Input: part model. Units: mm. Frame: model coordinates. Coordinates: 2 decimals unless noted, no trailing zeros. Loops run counter-clockwise (first coordinate to the right, second up) from the corner with the lowest first, then second, coordinate; pieces in that order, holes last.
```python
from build123d import *

# Parameters (mm, degrees)
SKETCH1_W                       = 558.8
SKETCH1_H                       = 25.4
BOSS_EXTRUDE1_DEPTH             = 6.35
F_1_4_0_25_DIAMETER_HOLE1_D     = 6.35
F_1_4_0_25_DIAMETER_HOLE1_DEPTH = 17.019524
F_1_4_0_25_DIAMETER_HOLE1_TIP   = 1.907732465
SKETCH5_R                       = 6.35
CUT_EXTRUDE1_DEPTH              = 280.760562803


with BuildPart() as part:
    # Sketch1 → Boss-Extrude1 (new body)
    with BuildSketch(Plane(origin=(0, 0, 0), x_dir=(1, 0, 0), z_dir=(0, 1, 0))):
        Rectangle(SKETCH1_W, SKETCH1_H)
    extrude(amount=BOSS_EXTRUDE1_DEPTH)

    # 1/4 (0.25) Diameter Hole1
    with Locations(Plane(origin=(0, 6.35, 0), x_dir=(1, 0, 0), z_dir=(0, 1, 0))):
        with Locations((-269.875, 0), (269.875, 0)):
            Hole(F_1_4_0_25_DIAMETER_HOLE1_D / 2, depth=F_1_4_0_25_DIAMETER_HOLE1_DEPTH)
            with Locations((0, 0, -(F_1_4_0_25_DIAMETER_HOLE1_DEPTH + F_1_4_0_25_DIAMETER_HOLE1_TIP / 2))):  # 118° drill point
                Cone(0, F_1_4_0_25_DIAMETER_HOLE1_D / 2, F_1_4_0_25_DIAMETER_HOLE1_TIP, mode=Mode.SUBTRACT)

    # Sketch5 → Cut-Extrude1 (cut, through all)
    with BuildSketch(Plane(origin=(0, 6.35, 0), x_dir=(1, 0, 0), z_dir=(0, 1, 0))):
        with Locations(Location((0, 0, 0), (0, 0, 270))):
            Circle(SKETCH5_R)
    extrude(amount=-CUT_EXTRUDE1_DEPTH, mode=Mode.SUBTRACT)


solid = part.part
```
Item 1: Section query A-A (x = 0). Output: boundary loops of the cut face in (y, z).
Result:
outline: (0, -12.7) - (6.35, -12.7) - (6.35, -6.35) - (0, -6.35) - close; (0, 6.35) - (6.35, 6.35) - (6.35, 12.7) - (0, 12.7) - close
Item 2: Line query: L1, parallel to X at y = 3, z = 5.5; L2, parallel to X at y = 1, z = -1; L3, parallel to X at y = 3.5, z = 4. Output: solid intervals per line, ascending.
Result:
L1: x = -279.4 to -3.17, 3.17 to 279.4
L2: x = -279.4 to -272.89, -266.86 to -6.27, 6.27 to 266.86, 272.89 to 279.4
L3: x = -279.4 to -4.93, 4.93 to 279.4
Item 3: Mould query, pull axis X, two halves, no side actions, for faces 1 (the face through (-3.86, 3.22, -5.04)), 2 (the face through (-3.9, 6.35, 5.5)). Classes: +X half, -X half, draft (parallel to the pull), parting line (faces both ways), or undercut.
Result:
face 1: undercut
face 2: draft
